For this review, take the finished solid that the model builds, in its own axes (mm). Give positions to 0.01 mm unless a question says otherwise; leave off trailing zeros. Order: outer loops, then holes, each group sorted by start corner. A loop starts at its lowest first (then second) coordinate and runs counter-clockwise, first axis right, second up.
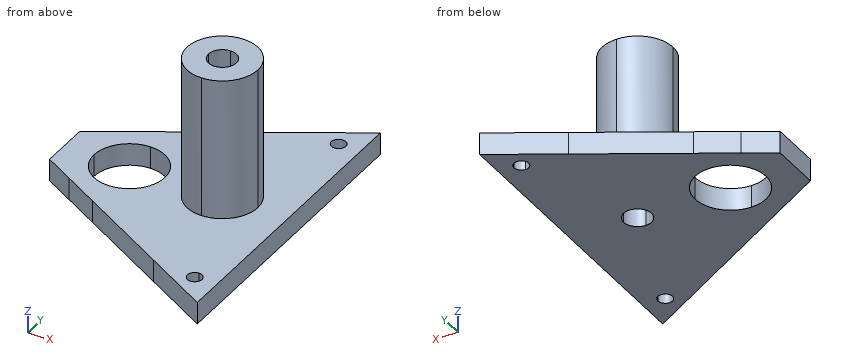
from build123d import *

# Parameters (mm, degrees)
F1_DEPTH = 5
F2_DEPTH = 37


with BuildPart() as f1:
    # F0 (on Top) → F1 (new body)
    with BuildSketch(Plane.XY):
        with BuildLine():
            Line((-3.35, 62.5), (0, 62.5))
            Line((0, 62.5), (0, 70))
            Line((0, 70), (-15, 61.3397447815))
            Line((-15, 61.3397447815), (-15, 43))
            ThreePointArc((-15, 43), (-9.3431457505, 40.6568542495), (-7, 35))
            Line((-7, 35), (-5, 35))
            Line((-5, 35), (-5, 60.85))
            ThreePointArc((-5, 60.85), (-6.166726189, 63.666726189), (-3.35, 62.5))
        make_face()
        with BuildLine():
            Line((-5, 35), (0, 35))
            Line((0, 35), (0, 62.5))
            Line((0, 62.5), (-3.35, 62.5))
            ThreePointArc((-3.35, 62.5), (-3.833273811, 61.333273811), (-5, 60.85))
            Line((-5, 60.85), (-5, 35))
        make_face()
        with BuildLine():
            Line((-3.35, 7.5), (0, 7.5))
            Line((0, 7.5), (0, 35))
            Line((0, 35), (-5, 35))
            Line((-5, 35), (-5, 9.15))
            ThreePointArc((-5, 9.15), (-3.833273811, 8.666726189), (-3.35, 7.5))
        make_face()
        with BuildLine():
            Line((-15, 8.6602552185), (0, 0))
            Line((0, 0), (0, 7.5))
            Line((0, 7.5), (-3.35, 7.5))
            ThreePointArc((-3.35, 7.5), (-6.166726189, 6.333273811), (-5, 9.15))
            Line((-5, 9.15), (-5, 35))
            Line((-5, 35), (-7, 35))
            ThreePointArc((-7, 35), (-9.3431457505, 29.3431457505), (-15, 27))
            Line((-15, 27), (-15, 8.6602552185))
        make_face()
        with BuildLine():
            Line((-36, 20.7846125245), (-15, 8.6602552185))
            Line((-15, 8.6602552185), (-15, 27))
            ThreePointArc((-15, 27), (-20.6568542495, 29.3431457505), (-23, 35))
            Line((-23, 35), (-28, 35))
            ThreePointArc((-28, 35), (-30.3431457505, 29.3431457505), (-36, 27))
            Line((-36, 27), (-36, 20.7846125245))
        make_face()
        with BuildLine():
            Line((-28, 35), (-23, 35))
            ThreePointArc((-23, 35), (-20.6568542495, 40.6568542495), (-15, 43))
            Line((-15, 43), (-15, 61.3397447815))
            Line((-15, 61.3397447815), (-36, 49.2153874755))
            Line((-36, 49.2153874755), (-36, 43))
            ThreePointArc((-36, 43), (-30.3431457505, 40.6568542495), (-28, 35))
        make_face()
        with BuildLine():
            Line((-44, 44.5965846923), (-44, 35))
            ThreePointArc((-44, 35), (-41.6568542495, 40.6568542495), (-36, 43))
            Line((-36, 43), (-36, 49.2153874755))
            Line((-36, 49.2153874755), (-44, 44.5965846923))
        make_face()
        with BuildLine():
            Line((-44, 25.4034153077), (-36, 20.7846125245))
            Line((-36, 20.7846125245), (-36, 27))
            ThreePointArc((-36, 27), (-41.6568542495, 29.3431457505), (-44, 35))
            Line((-44, 35), (-44, 25.4034153077))
        make_face()
        Polygon((-50.62177, 29.226496521), (-44, 25.4034153077), (-44, 35), (-50.62177, 35), align=None)
        Polygon((-50.62177, 35), (-44, 35), (-44, 44.5965846923), (-50.62177, 40.773503479), align=None)
    extrude(amount=F1_DEPTH)

    # F0 (on Top) → F2 (join)
    with BuildSketch(Plane.XY):
        with BuildLine():
            ThreePointArc((-15, 43), (-20.6568542495, 40.6568542495), (-23, 35))
            Line((-23, 35), (-18.15, 35))
            ThreePointArc((-18.15, 35), (-17.2273863607, 37.2273863607), (-15, 38.15))
            Line((-15, 38.15), (-15, 43))
        make_face()
        with BuildLine():
            Line((-11.85, 35), (-7, 35))
            ThreePointArc((-7, 35), (-9.3431457505, 40.6568542495), (-15, 43))
            Line((-15, 43), (-15, 38.15))
            ThreePointArc((-15, 38.15), (-12.7726136393, 37.2273863607), (-11.85, 35))
        make_face()
        with BuildLine():
            Line((-15, 31.85), (-15, 27))
            ThreePointArc((-15, 27), (-9.3431457505, 29.3431457505), (-7, 35))
            Line((-7, 35), (-11.85, 35))
            ThreePointArc((-11.85, 35), (-12.7726136393, 32.7726136393), (-15, 31.85))
        make_face()
        with BuildLine():
            ThreePointArc((-23, 35), (-20.6568542495, 29.3431457505), (-15, 27))
            Line((-15, 27), (-15, 31.85))
            ThreePointArc((-15, 31.85), (-17.2273863607, 32.7726136393), (-18.15, 35))
            Line((-18.15, 35), (-23, 35))
        make_face()
    extrude(amount=F2_DEPTH)


solid = f1.part
1) We need section D-D on x = -42. Give the boundary of the cut face in (y, z), then the cut area to 3 significant figures.
Answer sheet:
outline: (24.25, 0) - (29.71, 0) - (29.71, 5) - (24.25, 5) - close; (40.29, 0) - (45.75, 0) - (45.75, 5) - (40.29, 5) - close
area: 54.6 mm2
2) Clearance check with flat-ended pins moving along their axes: pin 1 (4 mm diameter, centred on x = -5, y = 7.5, fed in from +Z); pin 2 (5 mm diameter, centred on y = 30, z = 32, fed in from +X); pin 3 (4 mm diameter, centred on x = -17, z = 23, fed in from -Y). State where each tip first meets the part, or that it passes through.
Answer sheet:
pin 1: stops at z = 5
pin 2: stops at x = -7.4
pin 3: stops at y = 27
3) We need section C-C on x = -8. Give the boundary of the cut face in (y, z).
Answer sheet:
outline: (4.62, 0) - (65.38, 0) - (65.38, 5) - (38.87, 5) - (38.87, 37) - (31.13, 37) - (31.13, 5) - (4.62, 5) - close
4) We need section A-A on z = 11. Give the boundary of the cut face in (x, y).
Answer sheet:
outline: circle Ø16 at (-15, 35); hole circle Ø6.3 at (-15, 35)
5) To check wall thickness, follow line 1 (Y direction, x = -5, z = 1); line 2 (Z direction, x = -18.5, y = 18.5); line 3 (X direction, y = 62.5, z = 1.9). State the ranges of each line that lie inside material, in increasing order.
Answer sheet:
line 1: y = 2.89 to 5.85, 9.15 to 60.85, 64.15 to 67.11
line 2: z = 0 to 5
line 3: x = -12.99 to -6.65, -3.35 to 0
6) We need section B-B on x = -16.5. Give the boundary of the cut face in (y, z), then the cut area to 3 significant figures.
Answer sheet:
outline: (9.53, 0) - (32.23, 0) - (32.23, 37) - (27.14, 37) - (27.14, 5) - (9.53, 5) - close; (37.77, 0) - (60.47, 0) - (60.47, 5) - (42.86, 5) - (42.86, 37) - (37.77, 37) - close
area: 553 mm2
